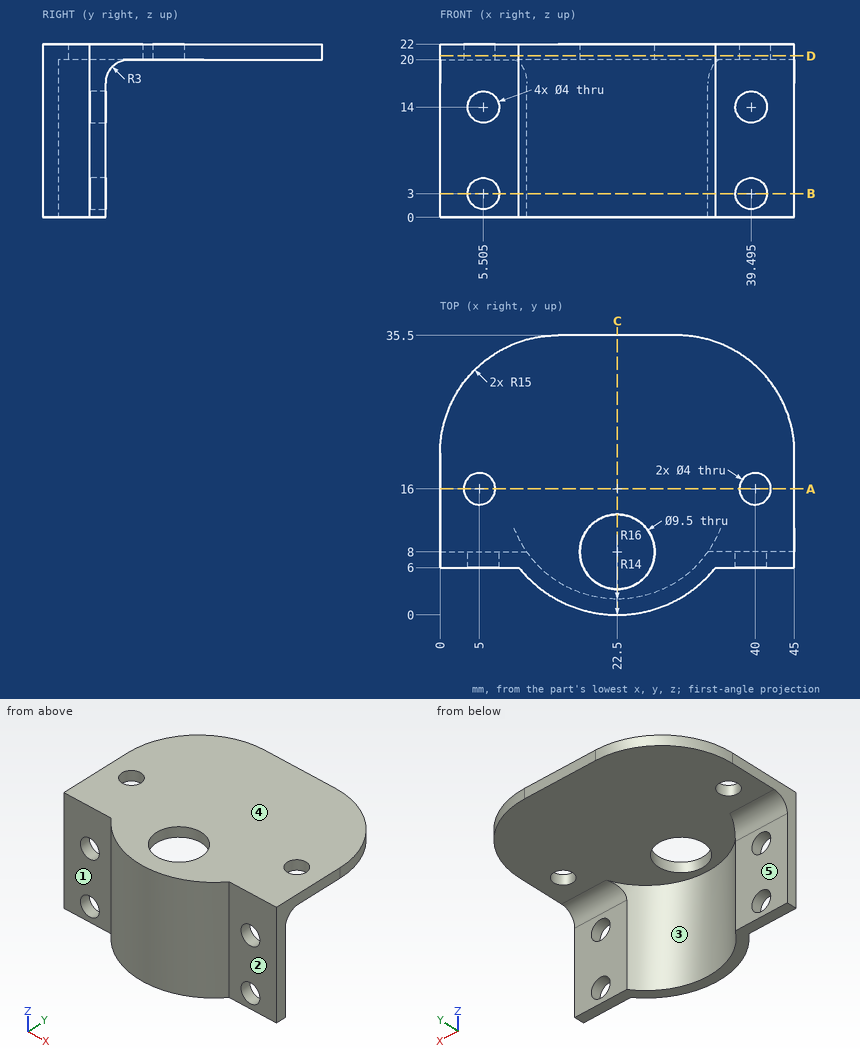
Here's the drawing with two shaded views (mm, measured from the low corner). I have some questions. A direction names the side the tool comes from. Coordinates: 2 decimals unless noted, no trailing zeros. Loops run counter-clockwise (first coordinate to the right, second up) from the corner with the lowest first, then second, coordinate; pieces in that order, holes last. Notation, with made-up numbers: M 33,64 L 58,64 A12 ccw 58,69 Z; hole C 89.25,65 d11. An arc over 180 degrees is marked long. Answer as CSV lines item,"result". Start each with the question number.
1. Suppose I cut it at D-D, the plane z = 20.5. List the corners of the cut face in (x, y) for me, plus the area to 3 significant figures.
2. Suppose I cut it at C-C, the plane x = 22.5. List the corners of the cut face in (y, z) for me.
3. For the marked faces 1, 2, 3, 4 and 5, which set-ups out of +Z, -Z, +X, -X, +Y, -Y let a thin tool reach every point of the face, with its end or its side?
4. If I drill on probe 1 along X at (y, z) = (8, 21.3); probe 2 along X at (y, z) = (7.4, 3) (1 decimal); probe 3 along Z at (x, y) = (12, 26), over which ranges is the centre line in solid material (lowest first)? Write a range as [from, to].
5. Suppose I cut it at A-A, the plane y = 16. List the corners of the cut face in (x, z) for me.
6. For pin 1 Ø4 at (x, z) = (13.5, 14) entering from +Y; pin 2 Ø12 at (x, z) = (4, 10.5) entering from +Y; pin 3 Ø6.5 at (x, z) = (5.51, 3) entering from -Y; pin 4 Ø12 at (y, z) = (12.5, 3.5) entering from -X, each with a flat end and sliding along its axis, tell me the tip position at first contact or that it passes through.
7. Suppose I cut it at B-B, the plane z = 3. List the corners of the cut face in (x, y) for me (1 decimal).
Output:
1,outline,"M 0,6 L 10.01,6 A16 ccw 34.99,6 L 45,6 L 45,20.5 A15 ccw 30,35.5 L 15,35.5 A15 ccw 0,20.5 Z; hole C 5,16 d4; hole C 22.5,8 d9.5; hole C 40,16 d4"
1,area,"1,240 mm^2"
2,outline,"M 0,0 L 2,0 L 2,20 L 3.25,20 L 3.25,22 L 0,22 Z; M 12.75,20 L 35.5,20 L 35.5,22 L 12.75,22 Z"
3,face 1,"+Z, -Z, -X, -Y"
3,face 2,"+Z, -Z, +X, -Y"
3,face 3,"-Z, +Y"
3,face 4,"+Z, +X, -X, +Y, -Y"
3,face 5,"-Z, +X, -X, +Y"
4,probe 1,"x = [0, 17.75], [27.25, 45]"
4,probe 2,"x = [0, 3.5], [7.5, 11.5], [33.5, 37.5], [41.5, 45]"
4,probe 3,"z = [20, 22]"
5,outline,"M 0,20 L 3,20 L 3,22 L 0,22 Z; M 7,20 L 38,20 L 38,22 L 7,22 Z; M 42,20 L 45,20 L 45,22 L 42,22 Z"
6,pin 1,"stops at y = 7.34"
6,pin 2,"stops at y = 8"
6,pin 3,"stops at y = 6"
6,pin 4,"stops at x = 0"
7,outline,"M 0,6 L 3.5,6 L 3.5,8 L 0,8 Z; M 7.5,6 L 10,6 A16 ccw 35,6 L 37.5,6 L 37.5,8 L 34,8 A14 cw 11,8 L 7.5,8 Z; M 41.5,6 L 45,6 L 45,8 L 41.5,8 Z"
